Autodesk Inventor part; units mm, degrees
ref_plane "YZ Plane" through (0, 0, 0) normal (1, 0, 0) x (0, 1, 0)
ref_plane "XZ Plane" through (0, 0, 0) normal (0, 1, 0) x (-1, 0, 0)
ref_plane "XY Plane" through (0, 0, 0) normal (0, 0, 1) x (1, 0, 0)
sketch "Sketch1" plane through (0, 0, 0) normal (0, 1, 0) x (-1, 0, 0)
  circle A0 centre (-36.9127, -68.2201) radius 2.1844
  circle A1 centre (39.2873, -68.2201) radius 2.1844
  arc A2 (39.2873, -74.5701) -> (45.6373, -68.2201) centre (39.2873, -68.2201) ccw
  arc A3 (-43.2627, -68.2201) -> (-36.9127, -74.5701) centre (-36.9127, -68.2201) ccw
  line L0 (39.2873, -74.5701) -> (-36.9127, -74.5701)
  line L1 (-43.2627, -68.2201) -> (-43.2627, 82.5924)
  line L2 (45.6373, -68.2201) -> (45.6373, 82.5924)
  line L3 (32.9373, 82.5924) -> (32.9373, -55.5201)
  line L4 (-30.5627, -55.5201) -> (-30.5627, 82.5924)
  line L5 (-32.1502, 84.1799) -> (-41.6752, 84.1799)
  line L6 (44.0498, 84.1799) -> (34.5248, 84.1799)
  arc A4 (45.6373, 82.5924) -> (44.0498, 84.1799) centre (44.0498, 82.5924) ccw
  arc A5 (34.5248, 84.1799) -> (32.9373, 82.5924) centre (34.5248, 82.5924) ccw
  arc A6 (-30.5627, 82.5924) -> (-32.1502, 84.1799) centre (-32.1502, 82.5924) ccw
  arc A7 (-41.6752, 84.1799) -> (-43.2627, 82.5924) centre (-41.6752, 82.5924) ccw
  line L7 (26.5873, -61.8701) -> (-24.2127, -61.8701)
  line L8 (32.9373, -55.5201) -> (26.5873, -61.8701)
  line L9 (-30.5627, -55.5201) -> (-24.2127, -61.8701)
  point P0 (0, 0)
  point P1 (-43.2627, 84.1799)
  point P2 (45.6373, 84.1799)
  point P3 (-30.5627, -61.8701)
  point P4 (32.9373, -61.8701)
  dimension "d0" = 152.4
  dimension "d1" = 152.4
  dimension "d2" = 1.5875
  dimension "d3" = 6.35
  dimension "d4" = 6.35
  dimension "d5" = 6.35
  dimension "d6" = 6.35
extrude "Extrusion1" add sketch "Sketch1" along normal blind 1.5875
properties part number "Ring Guard" material "Acetal Resin, White"
Could you check a few things on this model? Use its own coordinates, in mm. A direction names the side the tool comes from. Give positions to 0.01 mm unless a question says otherwise; leave off trailing zeros. Write each loop counter-clockwise with the first axis right and the second up, starting at its lowest first coordinate (ties: lowest second). Pieces come first, ordered by that corner, then holes. Notation, with made-up numbers: (-3.75, 38.5) - (44.25, 38.5) arc R9 cw to (44.25, 50.5) - close; hole circle Ø6 at (23, 48.5). An arc over 180 degrees is marked (long way). Use CSV: the item, a comma, the result in double quotes. Start each with the question number.
Item 1: I want a section at D-D, the plane x = 28. Please give me the cut outline in (y, z).
Item 2: If I drill on line 1 along X through (y, z) = (0.2, -7); line 2 along Z through (x, y) = (-23, 1); line 3 along Z through (x, y) = (32, 1.5), over which ranges is the centre line in solid material (lowest first)?
Item 3: I want a section at B-B, the plane y = 1.3. Give the number of separate pieces and of enclosed holes in the cut face, then the cut area to 3 significant figures.
Item 4: If we mould it in two halves opening along X, with no side actions, what happens to faces 3 (the face through (41.35, 0.78, -72.76)), 4 (the face through (32, 1.588, -12)), 5 (the face through (35.905, 0.783, -66.282))? For each: pulls with the +X half, pulls with the -X half, needs draft (parallel to the pull), parting line crosses it, or undercut.
Item 5: For faces 1 (the face through (32, 0, -12)), 2 (the face through (27.43, 0.78, -58.65)), which set-ups out of +Z, -Z, +X, -X, +Y, -Y let a thin tool reach every point of the face, with its end or its side?
Item 6: I want a section at C-C, the plane x = -2.5. Please give me the cut outline in (y, z), then the cut area to 3 significant figures.
Item 7: I want a section at A-A, the plane z = 44. Please give me the cut outline in (x, y), then the cut area to 3 significant figures.
Findings:
1,outline,"(0, -74.57) - (1.59, -74.57) - (1.59, -58.08) - (0, -58.08) - close"
2,line 1,"x = -45.64 to -32.94, 30.56 to 43.26"
2,line 2,"z = -74.57 to -61.87"
2,line 3,"z = -74.57 to 84.17"
3,separate pieces,"1"
3,enclosed holes,"2"
3,area,"4,830 mm2"
4,face 3,"pulls with the +X half"
4,face 4,"needs draft"
4,face 5,"undercut"
5,face 1,"+Z, -Z, +X, -X, -Y"
5,face 2,"+Z, +Y, -Y"
6,outline,"(0, -74.57) - (1.59, -74.57) - (1.59, -61.87) - (0, -61.87) - close"
6,area,"20.2 mm2"
7,outline,"(-45.64, 0) - (-32.94, 0) - (-32.94, 1.59) - (-45.64, 1.59) - close; (30.56, 0) - (43.26, 0) - (43.26, 1.59) - (30.56, 1.59) - close"
7,area,"40.3 mm2"
